```python
from build123d import *

# Parameters (mm, degrees)
F0_W     = 80
F0_H     = 16
F1_DEPTH = 9
F2_R     = 2.5
F3_DEPTH = 2
F4_W     = 77
F4_H     = 13
F4_R     = 3.25
F4_R_2   = 2.5
F5_DEPTH = 8
F6_R     = 1.25
F7_DEPTH = 10


with BuildPart() as f1:
    # F0 (on Top) → F1 (new body)
    with BuildSketch(Plane.XY):
        Rectangle(F0_W, F0_H)
    extrude(amount=F1_DEPTH)

    # F2 (on face) → F3 (join)
    with BuildSketch(Plane.XY.offset(9)):
        with Locations((-36, 4)):
            Circle(F2_R)
        with Locations((-36, -4)):
            Circle(F2_R)
        with Locations((-28, 4)):
            Circle(F2_R)
        with Locations((-28, -4)):
            Circle(F2_R)
        with Locations((-20, 4)):
            Circle(F2_R)
        with Locations((-20, -4)):
            Circle(F2_R)
        with Locations((-12, 4)):
            Circle(F2_R)
        with Locations((-12, -4)):
            Circle(F2_R)
        with Locations((-4, 4)):
            Circle(F2_R)
        with Locations((-4, -4)):
            Circle(F2_R)
        with Locations((4, 4)):
            Circle(F2_R)
        with Locations((4, -4)):
            Circle(F2_R)
        with Locations((12, 4)):
            Circle(F2_R)
        with Locations((12, -4)):
            Circle(F2_R)
        with Locations((20, 4)):
            Circle(F2_R)
        with Locations((20, -4)):
            Circle(F2_R)
        with Locations((28, 4)):
            Circle(F2_R)
        with Locations((28, -4)):
            Circle(F2_R)
        with Locations((36, 4)):
            Circle(F2_R)
        with Locations((36, -4)):
            Circle(F2_R)
    extrude(amount=F3_DEPTH)

    # F4 (on face) → F5 (cut)
    with BuildSketch(Plane(origin=(0, 0, 0), x_dir=(1, 0, 0), z_dir=(0, 0, -1))):
        Rectangle(F4_W, F4_H)
        with Locations((-32, 0)):
            Circle(F4_R, mode=Mode.SUBTRACT)
        with Locations((-24, 0)):
            Circle(F4_R, mode=Mode.SUBTRACT)
        with Locations((-16, 0)):
            Circle(F4_R, mode=Mode.SUBTRACT)
        with Locations((-8, 0)):
            Circle(F4_R, mode=Mode.SUBTRACT)
        Circle(F4_R, mode=Mode.SUBTRACT)
        with Locations((8, 0)):
            Circle(F4_R, mode=Mode.SUBTRACT)
        with Locations((16, 0)):
            Circle(F4_R, mode=Mode.SUBTRACT)
        with Locations((24, 0)):
            Circle(F4_R, mode=Mode.SUBTRACT)
        with Locations((32, 0)):
            Circle(F4_R, mode=Mode.SUBTRACT)
        with Locations((-32, 0)):
            Circle(F4_R_2)
        with Locations((-24, 0)):
            Circle(F4_R_2)
        with Locations((-16, 0)):
            Circle(F4_R_2)
        with Locations((-8, 0)):
            Circle(F4_R_2)
        Circle(F4_R_2)
        with Locations((8, 0)):
            Circle(F4_R_2)
        with Locations((16, 0)):
            Circle(F4_R_2)
        with Locations((24, 0)):
            Circle(F4_R_2)
        with Locations((32, 0)):
            Circle(F4_R_2)
    extrude(amount=-F5_DEPTH, mode=Mode.SUBTRACT)

    # F6 (on face) → F7 (cut)
    with BuildSketch(Plane(origin=(0, 0, 0), x_dir=(1, 0, 0), z_dir=(0, 0, -1))):
        with Locations((-36, 4)):
            Circle(F6_R)
        with Locations((-36, -4)):
            Circle(F6_R)
        with Locations((-28, 4)):
            Circle(F6_R)
        with Locations((-28, -4)):
            Circle(F6_R)
        with Locations((-20, 4)):
            Circle(F6_R)
        with Locations((-20, -4)):
            Circle(F6_R)
        with Locations((-12, 4)):
            Circle(F6_R)
        with Locations((-12, -4)):
            Circle(F6_R)
        with Locations((-4, 4)):
            Circle(F6_R)
        with Locations((-4, -4)):
            Circle(F6_R)
        with Locations((4, 4)):
            Circle(F6_R)
        with Locations((4, -4)):
            Circle(F6_R)
        with Locations((12, 4)):
            Circle(F6_R)
        with Locations((12, -4)):
            Circle(F6_R)
        with Locations((20, 4)):
            Circle(F6_R)
        with Locations((20, -4)):
            Circle(F6_R)
        with Locations((28, 4)):
            Circle(F6_R)
        with Locations((28, -4)):
            Circle(F6_R)
        with Locations((36, 4)):
            Circle(F6_R)
        with Locations((36, -4)):
            Circle(F6_R)
    extrude(amount=-F7_DEPTH, mode=Mode.SUBTRACT)


solid = f1.part
```
Design review of the part built by this model. Coordinates are the model's own, in mm. A direction names the side the tool comes from. Coordinates: 2 decimals unless noted, no trailing zeros. Order: outer loops, then holes, each group sorted by start corner. A loop starts at its lowest first (then second) coordinate and runs counter-clockwise, first axis right, second up.
1) Wall thickness on line 1 along Y through (x, z) = (12, 9.4); line 2 along Y through (x, z) = (-24, 1.75); line 3 along Y through (x, z) = (-28, 8.45): over which ranges is each line inside the solid? List them lowest first.
2) Take a section at B-B, the plane x = 16. Give the boundary of the cut face in (y, z), and give its area (3 significant figures).
3) Take a section at C-C, the plane x = -12. Give the boundary of the cut face in (y, z), and give its area (3 significant figures).
4) Clearance check with flat-ended pins moving along their axes: pin 1 (3 mm diameter, centred on x = -28, y = 4, fed in from -Z); pin 2 (6.5 mm diameter, centred on x = -8, y = 0, fed in from +Z); pin 3 (2 mm diameter, centred on x = -12, y = -4, fed in from -Z). State where each tip first meets the part, or that it passes through.
5) Take a section at A-A, the plane z = 1. State how many separate pieces and enclosed holes the cut face has, and give its area (3 significant figures).
6) For faces 1 (the flat face through (-36, -4, 10)), 2 (the cylindrical face through (-29.84, -2.31, 9.99)), 3 (the flat face through (-20, 4, 11)), list the 3-axis set-ups (+Z, -Z, +X, -X, +Y, -Y) from which the entire face can be reached by the end or side of a thin tool; tool diameter is ignored.
7) Mouldability with a two-part tool opening along X and no side actions: class faces 4 (the cylindrical face through (-26.5, -0.1, 3.9)), 5 (the flat face through (4, 4, 11)) as +X half, -X half, draft (parallel to the pull), parting line (faces both ways), or undercut.
Returned:
1. line 1: y = -6.5 to -5.25, -2.75 to -1.5, 1.5 to 2.75, 5.25 to 6.5
1. line 2: y = -8 to -6.5, -3.25 to -2.5, 2.5 to 3.25, 6.5 to 8
1. line 3: y = -8 to -5.25, -2.75 to 2.75, 5.25 to 8
2. outline: (-8, 0) - (-6.5, 0) - (-6.5, 8) - (-3.25, 8) - (-3.25, 0) - (-2.5, 0) - (-2.5, 8) - (2.5, 8) - (2.5, 0) - (3.25, 0) - (3.25, 8) - (6.5, 8) - (6.5, 0) - (8, 0) - (8, 9) - (-8, 9) - close
2. area: 52.0 mm2
3. outline: (-8, 0) - (-6.5, 0) - (-6.5, 8) - (-5.25, 8) - (-5.25, 10) - (-2.75, 10) - (-2.75, 8) - (2.75, 8) - (2.75, 10) - (5.25, 10) - (5.25, 8) - (6.5, 8) - (6.5, 0) - (8, 0) - (8, 9) - (6.5, 9) - (6.5, 11) - (1.5, 11) - (1.5, 9) - (-1.5, 9) - (-1.5, 11) - (-6.5, 11) - (-6.5, 9) - (-8, 9) - close
3. area: 50.0 mm2
4. pin 1: stops at z = 8
4. pin 2: stops at z = 11
4. pin 3: stops at z = 10
5. separate pieces: 10
5. enclosed holes: 10
5. area: 401 mm2
6. face 1: -Z
6. face 2: +Z
6. face 3: +Z, +X, -X, +Y, -Y
7. face 4: undercut
7. face 5: draft
